```python
from build123d import *

# Parameters (mm, degrees)
FILLET1_R = 10


with BuildPart() as part:
    # Sketch1 → Revolve1 (revolve)
    with BuildSketch(Plane.XY):
        with BuildLine():
            Line((0, 0), (1.5, 0))
            Line((1.5, 0), (1.5, -2.5))
            Line((1.5, -2.5), (1.3, -5))
            Line((1.3, -5), (1.3, -38.480131585))
            ThreePointArc((1.3, -38.480131585), (1.876131236, -40.69291528), (0, -42))
            Line((0, -42), (0, 0))
        make_face()
    revolve(axis=Axis((0, -119.770062165, 0), (0, 1, 0)))

    # Fillet1
    # the kernel refuses this fillet: 10 mm, written as the material it adds along each edge
    with BuildSketch(Plane(origin=(0, -5, 0), x_dir=(1, 0, 0), z_dir=(0, 0, 1))) as fillet1_piece_1:
        with BuildLine():
            CenterArc((1.3 + FILLET1_R, -FILLET1_R * 0.0399362039845), FILLET1_R, 175.42607874, 4.57392126)
            Line((1.3, -FILLET1_R * 0.0399362039845), (1.3, 0))
            Line((1.3, 0), (1.3 + FILLET1_R * 0.00318472146388, FILLET1_R * 0.0398090182984))
        make_face()
    revolve(axis=Axis((0, -5, 0), (0, 1, 0)))
    # the kernel refuses this fillet: 10 mm, written as the material it takes off along each edge
    with BuildSketch(Plane(origin=(0, -2.5, 0), x_dir=(1, 0, 0), z_dir=(0, 0, 1))) as fillet1_2_piece_1:
        with BuildLine():
            CenterArc((1.5 - FILLET1_R, FILLET1_R * 0.0399362039845), FILLET1_R, 355.42607874, 4.57392126)
            Line((1.5 - FILLET1_R * 0.00318472146387, -FILLET1_R * 0.0398090182984), (1.5, 0))
            Line((1.5, 0), (1.5, FILLET1_R * 0.0399362039845))
        make_face()
    revolve(axis=Axis((0, -2.5, 0), (0, 1, 0)), mode=Mode.SUBTRACT)


solid = part.part
```
Here's how the part is built. I have some questions about the finished solid (model axes, mm). Give positions to 0.01 mm unless a question says otherwise; leave off trailing zeros. Loops run counter-clockwise (first coordinate to the right, second up) from the corner with the lowest first, then second, coordinate; pieces in that order, holes last. Notation, with made-up numbers: M 64,17 L 122,17 A21 ccw 122,43 Z; hole C 10.5,36 d1. An arc over 180 degrees is marked long. Return JSON: item names as keys, results as strings.
Item 1: Please list where these lines run through material, in increasing order: line 1 (Z direction, x = -0.1, y = -27.5); line 2 (X direction, y = -7, z = 1.05); line 3 (Y direction, x = 0.4, z = 1).
A:
{"line 1": "z = -1.3 to 1.3", "line 2": "x = -0.77 to 0.77", "line 3": "y = -41.69 to 0"}
Item 2: Imagine slicing it at A-A on y = -6.5. List the corners of the cut face in (x, z) for me.
A:
{"outline": "C 0,0 d2.6"}
Item 3: Thinking about a two-plate mould opening in Y: for faces 1 (the cylindrical face through (-0.17, -22.17, -1.29)), 2 (the cylindrical face through (-1.5, -1.07, -0.07)), 3 (the flat face through (0, 0, 0)), which applies, released by +Y, released by -Y, zero draft, split by the parting line, or undercut?
A:
{"face 1": "undercut", "face 2": "zero draft", "face 3": "released by +Y"}
Item 4: I'm going to push flat-ended pins straight in: pin 1 Ø1.5 at (y, z) = (-23, 0) entering from +X; pin 2 Ø2 at (x, y) = (0.5, -9) entering from +Z; pin 3 Ø2 at (x, y) = (0, -27) entering from -Z. Where does each tip first touch, or does it pass through?
A:
{"pin 1": "stops at x = 1.3", "pin 2": "stops at z = 1.3", "pin 3": "stops at z = -1.3"}
